Check sheet for the modelled part. Datum: model origin and axes. Units: mm. Face numbers are marked on the shaded views. A direction names the side the tool comes from. Coordinates: 2 decimals unless noted, no trailing zeros. Order: outer loops, then holes, each group sorted by start corner. A loop starts at its lowest first (then second) coordinate and runs counter-clockwise, first axis right, second up.
1. Cross-section at B-B (x = 3). Enter the section's corners in (y, z).
2. Cross-section at A-A (y = 1). Enter the section's corners in (x, z), then the cut area to 3 significant figures.
3. Thickness scan on line 1 (Y direction, x = 33, z = 12.25); line 2 (Z direction, x = 13.5, y = -1); line 3 (X direction, y = -19.5, z = 16). Record the ranges inside material, lowest first.
4. Set-up check for the marked faces 1, 2, 3 and 4: record each of +Z, -Z, +X, -X, +Y, -Y from which the full face is reachable in a straight line by a thin tool's end or side.
5. Cross-section at C-C (y = -31). Enter the section's corners in (x, z).
6. Cross-section at D-D (z = 18). Enter the section's corners in (x, y).
7. Gauge pin test, flat ends, axial feed: pin 1 Ø4 at (x, y) = (-10.49, -15.79) entering from +Z; pin 2 Ø4.5 at (x, z) = (32.5, 19.5) entering from +Y; pin 3 Ø12 at (y, z) = (-18, 20.5) entering from -X. Record the tip position at first contact, or that the pin passes through.
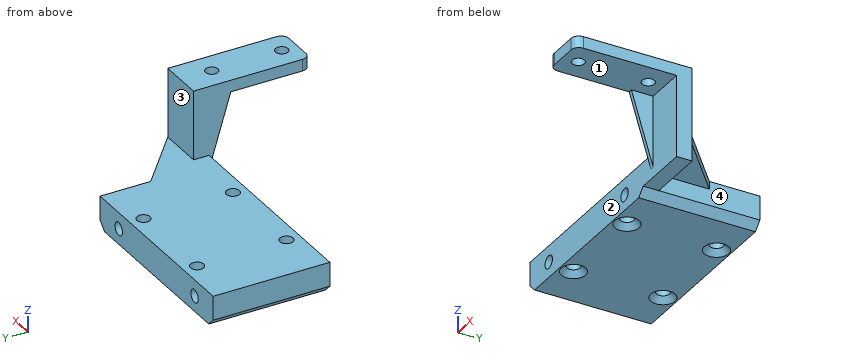
```python
from build123d import *

# Parameters (mm, degrees)
SKETCH_1_W                   = 50.7
SKETCH_1_H                   = 30
EXTRUDE_1_DEPTH              = 8.2
CUT_EXTRUDE_1_DEPTH          = 31
HOLE_WIZARD_M3_1_D           = 3.4
HOLE_WIZARD_M3_1_CSINK_D     = 6.3
HOLE_WIZARD_M3_1_CSINK_ANGLE = 90
SKETCH_5_R                   = 1.65
CUT_EXTRUDE_2_DEPTH          = 31
SKETCH_6_W                   = 6.2
SKETCH_6_H                   = 5
EXTRUDE_2_DEPTH              = 15
SKETCH_9_W                   = 11.54
SKETCH_9_H                   = 5
EXTRUDE_7_DEPTH              = 17.8
SKETCH_10_W                  = 11.54
SKETCH_10_H                  = 3
EXTRUDE_8_DEPTH              = 26
SKETCH_11_R                  = 1.6
CUT_EXTRUDE_3_DEPTH          = 4
EXTRUDE_10_DEPTH             = 1
FILLET_1_R                   = 2
CUT_EXTRUDE_4_DEPTH          = 1
EXTRUDE_11_DEPTH             = 2


with BuildPart() as part:
    # 草图1 → 凸台-拉伸1 (new body)
    with BuildSketch(Plane.XY):
        with Locations((1.504794521, -4.292808219)):
            Rectangle(SKETCH_1_W, SKETCH_1_H)
    extrude(amount=EXTRUDE_1_DEPTH)

    # 草图2 → 切除-拉伸1 (cut, through all)
    with BuildSketch(Plane(origin=(0, 10.707191781, 0), x_dir=(1, 0, 0), z_dir=(0, 1, 0))):
        Polygon((-21.845205479, 0), (-23.845205479, -2), (-23.845205479, 0), align=None)
        Polygon((24.854794521, 0), (26.854794521, -2), (26.854794521, 0), align=None)
    extrude(amount=-CUT_EXTRUDE_1_DEPTH, mode=Mode.SUBTRACT)

    # M3 平头机械螺钉的锥形沉头孔1 (through all)
    with Locations(Plane(origin=(-10.486055507, -15.792808219, 0), x_dir=(-1, 0, 0), z_dir=(0, 0, -1))):
        with Locations((0, 0), (-23.990850028, 0), (-23.990850028, 23), (0.009149972, 23)):
            CounterSinkHole(HOLE_WIZARD_M3_1_D / 2, HOLE_WIZARD_M3_1_CSINK_D / 2, counter_sink_angle=HOLE_WIZARD_M3_1_CSINK_ANGLE)

    # 草图5 → 切除-拉伸2 (cut, through all)
    with BuildSketch(Plane.XZ.offset(19.292808219)):
        with Locations((-15.495205479, 4)):
            Circle(SKETCH_5_R)
        with Locations((18.504794521, 4)):
            Circle(SKETCH_5_R)
    extrude(amount=-CUT_EXTRUDE_2_DEPTH, mode=Mode.SUBTRACT)

    # 草图6 → 凸台-拉伸2 (add)
    with BuildSketch(Plane(origin=(26.854794521, 0, 0), x_dir=(0, 0, -1), z_dir=(1, 0, 0))):
        with Locations((-5.1, -16.792808219)):
            Rectangle(SKETCH_6_W, SKETCH_6_H)
    extrude(amount=EXTRUDE_2_DEPTH)

    # 草图9 → 凸台-拉伸7 (add)
    with BuildSketch(Plane.XY.offset(8.2)):
        with Locations((36.084794521, -16.792808219)):
            Rectangle(SKETCH_9_W, SKETCH_9_H)
    extrude(amount=EXTRUDE_7_DEPTH)

    # 草图10 → 凸台-拉伸8 (add)
    with BuildSketch(Plane.XZ.offset(19.292808219)):
        with Locations((36.084794521, 24.5)):
            Rectangle(SKETCH_10_W, SKETCH_10_H)
    extrude(amount=EXTRUDE_8_DEPTH)

    # 草图11 → 切除-拉伸3 (cut, through all)
    with BuildSketch(Plane(origin=(0, 0, 23), x_dir=(-1, 0, 0), z_dir=(0, 0, -1))):
        with Locations((-36.084794521, -41.292808219)):
            Circle(SKETCH_11_R)
        with Locations((-36.084794521, -23.292808219)):
            Circle(SKETCH_11_R)
    extrude(amount=-CUT_EXTRUDE_3_DEPTH, mode=Mode.SUBTRACT)

    # 草图15 → 凸台-拉伸10 (add)
    with BuildSketch(Plane.ZY.offset(-30.314794521)):
        Polygon((23, -24.883219003), (4.647869492, -19.292808219), (23, -19.292808219), align=None)
    extrude(amount=-EXTRUDE_10_DEPTH)

    # 圆角1
    fillet_1_edges = [part.edges().sort_by_distance(p)[0] for p in [
        (30.314794521, -45.292808219, 24.5),
        (41.854794521, -45.292808219, 24.5),
    ]]
    fillet(fillet_1_edges, radius=FILLET_1_R)

    # 草图17 → 切除-拉伸4 (cut)
    with BuildSketch(Plane(origin=(0, -14.292808219, 0), x_dir=(1, 0, 0), z_dir=(0, 1, 0))):
        Polygon((26.854794521, -8.2), (30.314794521, -8.2), (30.314794521, -26), (41.854794521, -26), (41.854794521, -2), (26.854794521, -2), align=None)
    extrude(amount=-CUT_EXTRUDE_4_DEPTH, mode=Mode.SUBTRACT)

    # 草图18 → 凸台-拉伸11 (add)
    with BuildSketch(Plane.XY.offset(8.2)):
        Polygon((26.854794521, -15.292808219), (30.314794521, -15.292808219), (41.854261071, -15.292808219), (26.854794521, -2.292808219), align=None)
    extrude(amount=-EXTRUDE_11_DEPTH)


solid = part.part
```
Data:
1. outline: (-19.29, 0) - (10.71, 0) - (10.71, 8.2) - (-19.29, 8.2) - close
2. outline: (-23.85, 2) - (-21.85, 0) - (24.85, 0) - (26.85, 2) - (26.85, 8.2) - (-23.85, 8.2) - close; hole circle Ø3.3 at (-15.5, 4); hole circle Ø3.3 at (18.5, 4)
2. area: 395 mm2
3. line 1: y = -19.29 to -15.29
3. line 2: z = 0 to 8.2
3. line 3: x = 30.31 to 31.31
4. face 1: -Z, +X, -Y
4. face 2: -Z, -Y
4. face 3: +X, +Y
4. face 4: -Z, +X, +Y
5. outline: (30.31, 23) - (41.85, 23) - (41.85, 26) - (30.31, 26) - close
6. outline: (30.31, -23.36) - (31.31, -23.36) - (31.31, -19.29) - (41.85, -19.29) - (41.85, -15.29) - (30.31, -15.29) - close
7. pin 1: stops at z = 8.2
7. pin 2: stops at y = -15.29
7. pin 3: stops at x = 30.31
